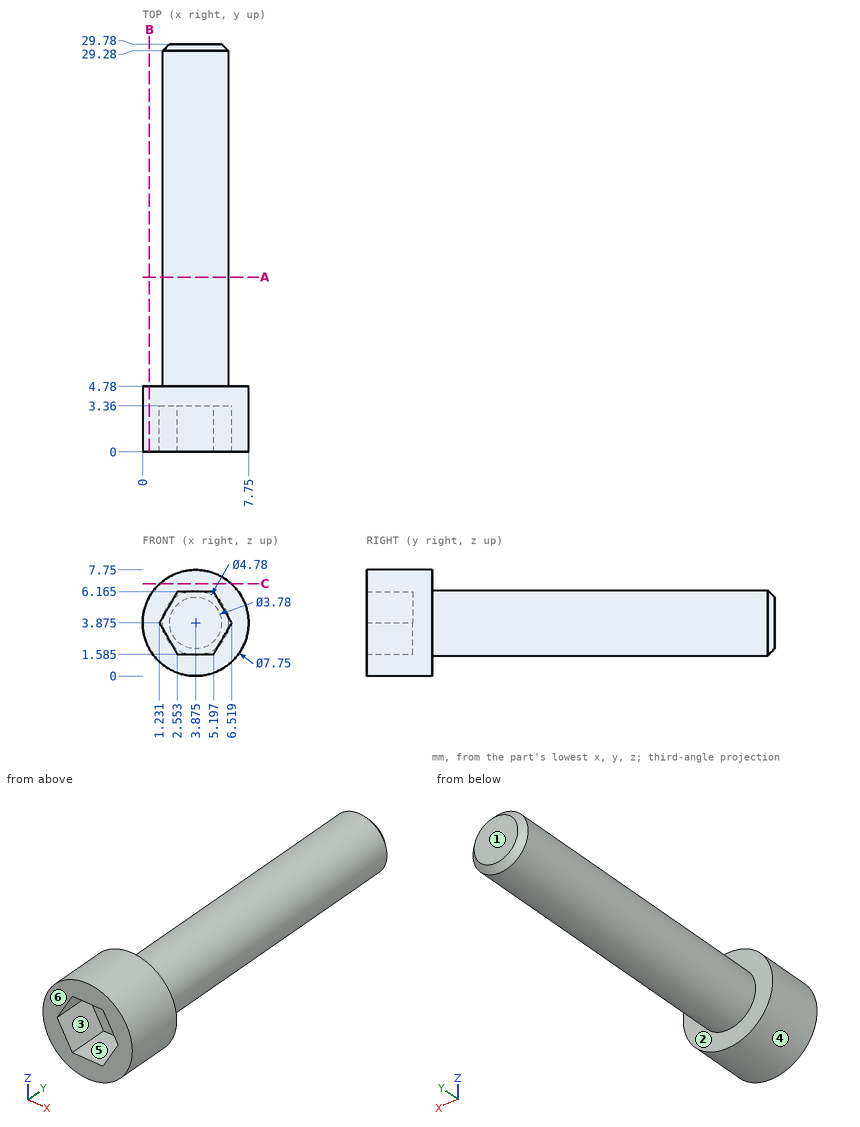
Design review of the part shown in the three views and the two pictorial views. Dimensions are in mm from the part's minimum x, y and z. A direction names the side the tool comes from. Coordinates: 2 decimals unless noted, no trailing zeros. Loops run counter-clockwise (first coordinate to the right, second up) from the corner with the lowest first, then second, coordinate; pieces in that order, holes last. Notation, with made-up numbers: (19, 45) - (46, 45) arc R29 ccw to (46, 73) - close; hole circle Ø9 at (41, 80). An arc over 180 degrees is marked (long way). Use a Markdown table: item, result. Add a question column.
Item 1: We need section C-C (z = 6.75). Give the boundary of the cut face in (x, y), and give its area (3 significant figures).
Item 2: Insertion check: pin 1 Ø3 at (x, y) = (1, 23.5) entering from +Z. The pin has a flat end and moves straight along its axis. Give the tip position at first contact, or say it passes through.
Item 3: We need section B-B (x = 0.5). Give the boundary of the cut face in (y, z), and give its area (3 significant figures).
Item 4: For line 1 (Z direction, x = 5, y = 3.25) (1 decimal); line 2 (Y direction, x = 2.5, z = 1.5); line 3 (Y direction, x = 5, z = 3.25), list the stretches that pass through material, from the lowest coordinate up.
Item 5: Tool access review of the marked faces 1, 2 and 3: name each direction out of +Z, -Z, +X, -X, +Y, -Y from which nothing blocks a thin tool from reaching the whole face with its end or side.
Item 6: Mouldability with a two-part tool opening along X and no side actions: class the marked faces 4, 5 and 6 as pulls with the +X half, pulls with the -X half, needs draft (parallel to the pull), parting line crosses it, or undercut.
Item 7: We need section A-A (y = 12.75). Give the boundary of the cut face in (x, z) (1 decimal).
Results list:
| question | item | result |
|---|---|---|
| 1 | outline | (1.28, 0) - (6.47, 0) - (6.47, 4.78) - (1.28, 4.78) - close |
| 1 | area | 24.8 mm^2 |
| 2 | pin 1 | stops at z = 5.83 |
| 3 | outline | (0, 1.97) - (4.78, 1.97) - (4.78, 5.78) - (0, 5.78) - close |
| 3 | area | 18.2 mm^2 |
| 4 | line 1 | z = 0.2 to 1.6, 6.2 to 7.6 |
| 4 | line 2 | y = 0 to 4.78 |
| 4 | line 3 | y = 3.36 to 29.78 |
| 5 | face 1 | +Z, -Z, +X, -X, +Y |
| 5 | face 2 | +Y |
| 5 | face 3 | -Y |
| 6 | face 4 | parting line crosses it |
| 6 | face 5 | undercut |
| 6 | face 6 | needs draft |
| 7 | outline | circle Ø4.8 at (3.9, 3.9) |
